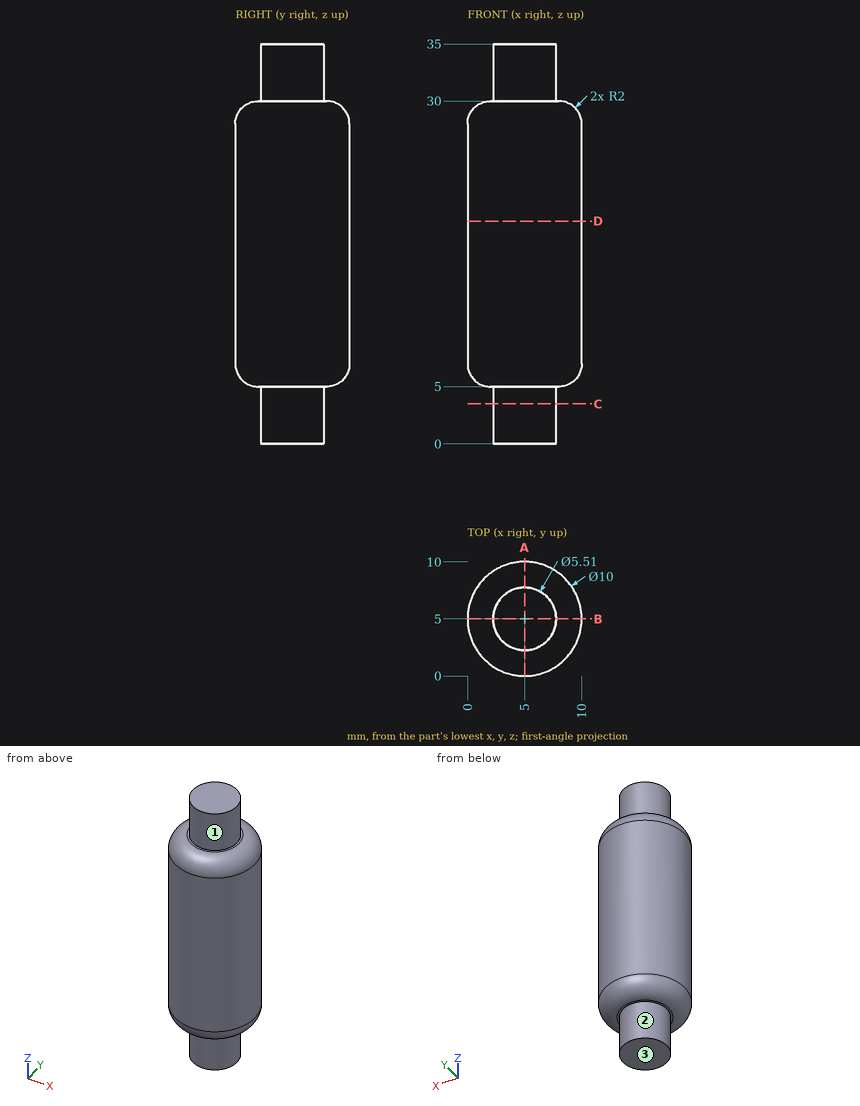
Could you check a few things on this drawing? It's one solid part, dimensions in mm from its lowest x, y, z. A direction names the side the tool comes from. Give positions to 0.01 mm unless a question says otherwise; leave off trailing zeros. Write each loop counter-clockwise with the first axis right and the second up, starting at its lowest first coordinate (ties: lowest second). Pieces come first, ordered by that corner, then holes. Notation, with made-up numbers: M 17.25,-22 L 63.25,-22 A29 ccw 63.25,10 Z; hole C -12,-36 d7. An arc over 180 degrees is marked long. Put each result on its own line as item: value. Start each with the question number.
Item 1: If we section it at C-C, the plane z = 3.5: Write out the boundary of the cut face in (x, y) (3 decimals).
Item 2: On a 3-axis mill with a long thin cutter (end or side, diameter ignored), from which of +Z, -Z, +X, -X, +Y, -Y can I reach the whole of each face in a straight line? I mean the marked faces 1, 2 and 3. Say none if no direction works.
Item 3: Will these pins go through, and if not, where does the flat tip stop? pin 1 (3 mm diameter, centred on x = 1.5, z = 9, fed in from -Y); pin 2 (3 mm diameter, centred on y = 3, z = 6, fed in from +X); pin 3 (5 mm diameter, centred on y = 9, z = 4.5, fed in from -X).
Item 4: If we section it at A-A, the plane x = 5: Write out the boundary of the cut face in (y, z) (3 decimals), then the cut area to 3 significant figures.
Item 5: I need wall thicknesses on L1, parallel to X at y = 5.25, z = 8.5; L2, parallel to X at y = 3.5, z = 32; L3, parallel to Y at x = 4.5, z = 14.5. Which ranges of each line are inside material? Lowest first, please. Write a range as from..to.
Item 6: If we section it at D-D, the plane z = 19.5: Write out the boundary of the cut face in (x, y).
Values:
1. outline: C 5,5 d5.51
2. face 1: +Z
2. face 2: -Z
2. face 3: -Z, +X, -X, +Y, -Y
3. pin 1: y = 0.42
3. pin 2: x = 9.94
3. pin 3: x = 0.68
4. outline: M 0,7 A2 ccw 2,5 L 2.245,5 L 2.245,0 L 7.755,0 L 7.755,5 L 8,5 A2 ccw 10,7 L 10,28 A2 ccw 8,30 L 7.755,30 L 7.755,35 L 2.245,35 L 2.245,30 L 2,30 A2 ccw 0,28 Z
4. area: 302 mm²
5. L1: 0.01..9.99
5. L2: 2.69..7.31
5. L3: 0.03..9.97
6. outline: C 5,5 d10
